For this review, use the dimensioned drawing (mm, ordinates from the lowest corner) and the shaded views. Coordinates: 2 decimals unless noted, no trailing zeros. Loops run counter-clockwise (first coordinate to the right, second up) from the corner with the lowest first, then second, coordinate; pieces in that order, holes last. Notation, with made-up numbers: (51.25, -5) - (55.25, -5) arc R17 ccw to (55.25, 19) - close; hole circle Ø3 at (-33, 52). An arc over 180 degrees is marked (long way). Answer in a Markdown table with one row per item. Add a question column.
(1) Clearance check with flat-ended pins moving along their axes: pin 1 (2 mm diameter, centred on y = 131, z = 2.5, fed in from +X); pin 2 (2 mm diameter, centred on y = 179.5, z = 1.5, fed in from -X); pin 3 (1.2 mm diameter, centred on x = 174.5, z = 2.5, fed in from -Y). State where each tip first meets the part, or that it passes through.
(2) We need section A-A, the plane y = 14. Write out the cut boundary in (x, z).
(3) We need section D-D, the plane y = 70. Write out the cut boundary in (x, z), plus the area to 3 significant figures.
(4) We need section B-B, the plane z = 0.75. Write out the cut boundary in (x, y), plus the area to 3 significant figures.
(5) To check wall thickness, follow L1, parallel to X at y = 42, z = 0.25 (1 decimal); L2, parallel to X at y = 174, z = 3.55 (1 decimal); L3, parallel to Y at x = 27, z = 3.55 (1 decimal). State the ranges of each line that lie inside material, in increasing order. Write a range as [from, to].
(6) We need section C-C, the plane x = 46.5. Write out the cut boundary in (y, z) (1 decimal), plus the area to 3 significant figures.
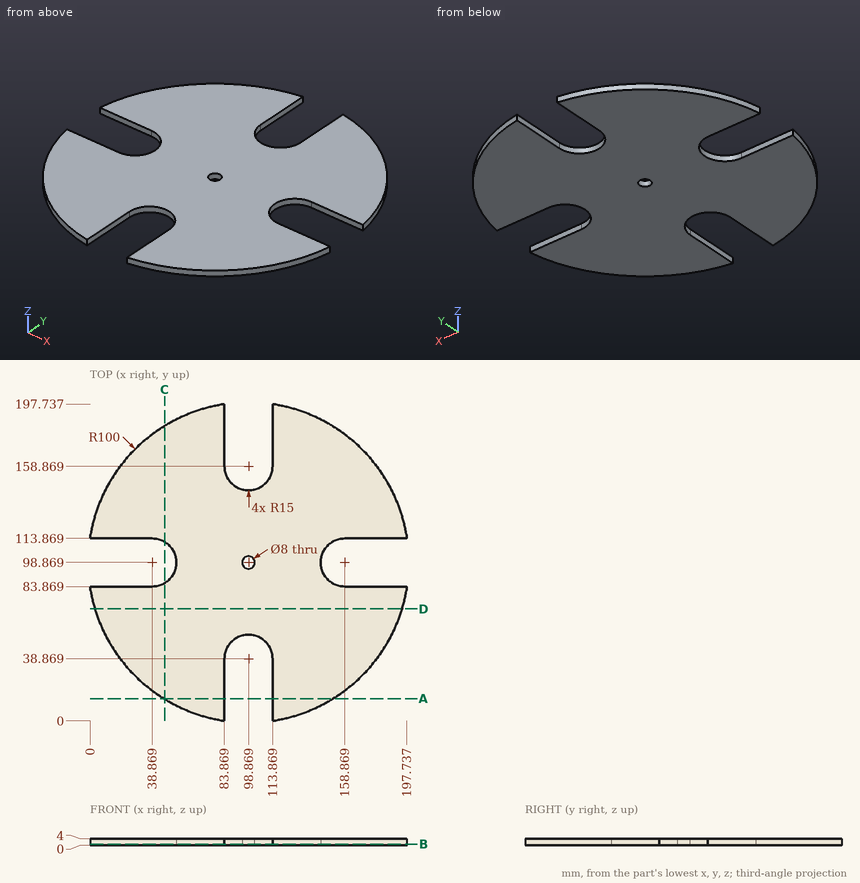
Responses:
| question | item | result |
|---|---|---|
| 1 | pin 1 | stops at x = 193.9 |
| 1 | pin 2 | stops at x = 38.38 |
| 1 | pin 3 | stops at y = 32.76 |
| 2 | outline | (45.98, 0) - (83.87, 0) - (83.87, 4) - (45.98, 4) - close; (113.87, 0) - (151.76, 0) - (151.76, 4) - (113.87, 4) - close |
| 3 | outline | (3.13, 0) - (194.61, 0) - (194.61, 4) - (3.13, 4) - close |
| 3 | area | 766 mm2 |
| 4 | outline | (0, 83.87) arc R100 ccw to (83.87, 0) - (83.87, 38.87) arc R15 cw to (113.87, 38.87) - (113.87, 0) arc R100 ccw to (197.74, 83.87) - (158.87, 83.87) arc R15 cw to (158.87, 113.87) - (197.74, 113.87) arc R100 ccw to (113.87, 197.74) - (113.87, 158.87) arc R15 cw to (83.87, 158.87) - (83.87, 197.74) arc R100 ccw to (0, 113.87) - (38.87, 113.87) arc R15 cw to (38.87, 83.87) - close; hole circle Ø8 at (98.87, 98.87) |
| 4 | area | 25,200 mm2 |
| 5 | L1 | x = [16.6, 84.2], [113.5, 181.1] |
| 5 | L2 | x = [32.9, 83.9], [113.9, 164.9] |
| 5 | L3 | y = [29.3, 83.9], [113.9, 168.4] |
| 6 | outline | (13.7, 0) - (86, 0) - (86, 4) - (13.7, 4) - close; (111.8, 0) - (184.1, 0) - (184.1, 4) - (111.8, 4) - close |
| 6 | area | 578 mm2 |
